Verification items for this drawing (mm, ordinates from the low corner). A direction names the side the tool comes from. Give positions to 0.01 mm unless a question says otherwise; leave off trailing zeros. Loops run counter-clockwise (first coordinate to the right, second up) from the corner with the lowest first, then second, coordinate; pieces in that order, holes last. Notation, with made-up numbers: (66, -20.75) -> (82, -20.75) arc R32 cw to (82, 13.25) -> close; hole circle Ø10 at (64.5, -32.75). An arc over 180 degrees is marked (long way). Answer as a JSON object with one key per item and string values.
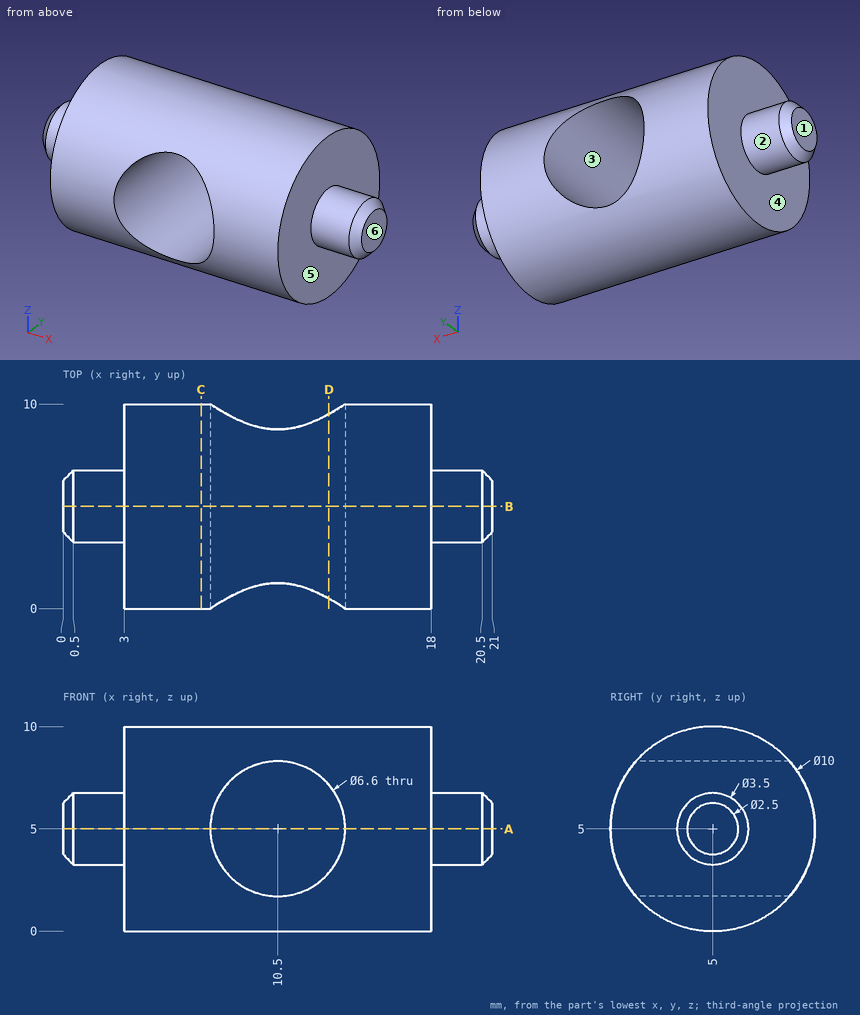
1) Section check C-C on x = 6.75. Record the cut outline in (y, z).
Geometry check:
{"outline": "circle Ø10 at (5, 5)"}
2) Draft check along Z on the marked faces 1, 2 and 3. Enter one of: pulls with the +Z half, pulls with the -Z half, needs draft (parallel to the pull), parting line crosses it, or undercut.
Geometry check:
{"face 1": "needs draft", "face 2": "parting line crosses it", "face 3": "undercut"}
3) Material ranges on line 1 along X through (y, z) = (6, 5); line 2 along X through (y, z) = (2.5, 5); line 3 along X through (y, z) = (5.25, 8.5), recorded low to high. Write a range as from..to.
Geometry check:
{"line 1": "x = 0..7.2, 13.8..21", "line 2": "x = 3..7.2, 13.8..18", "line 3": "x = 3..18"}
4) Section check D-D on x = 13. Record the cut outline in (y, z), plus the area to 3 significant figures.
Geometry check:
{"outline": "(0.49, 2.85) arc R5 ccw to (9.51, 2.85) -> close; (0.49, 7.15) -> (9.51, 7.15) arc R5 ccw to start", "area": "36.8 mm2"}
5) Section check A-A on z = 5. Record the cut outline in (x, y), plus the area to 4 significant figures.
Geometry check:
{"outline": "(0, 3.75) -> (0.5, 3.25) -> (3, 3.25) -> (3, 0) -> (7.2, 0) -> (7.2, 10) -> (3, 10) -> (3, 6.75) -> (0.5, 6.75) -> (0, 6.25) -> close; (13.8, 0) -> (18, 0) -> (18, 3.25) -> (20.5, 3.25) -> (21, 3.75) -> (21, 6.25) -> (20.5, 6.75) -> (18, 6.75) -> (18, 10) -> (13.8, 10) -> close", "area": "104.5 mm2"}
6) Tool access check on the marked faces 4, 5 and 6. Record the directions out of +Z, -Z, +X, -X, +Y, -Y that give a thin tool (end or side, any length) a straight path to the whole face; none if there is none.
Geometry check:
{"face 4": "-X", "face 5": "+X", "face 6": "+Z, -Z, +X, +Y, -Y"}
7) Depth check by flat-ended pin: P1, Ø4, axis at y = 1, z = 6, coming from the -X side; P2, Ø1.5, axis at x = 9, y = 2, coming from the +Z side; P3, Ø1, axis at x = 15, z = 2, coming from the +Y side. Enter the tip coordinate at first touch or a pass-through.
Geometry check:
{"P1": "stops at x = 3", "P2": "stops at z = 9.47", "P3": "stops at y = 9.33"}
8) Section check B-B on y = 5. Record the cut outline in (x, z).
Geometry check:
{"outline": "(0, 3.75) -> (0.5, 3.25) -> (3, 3.25) -> (3, 0) -> (18, 0) -> (18, 3.25) -> (20.5, 3.25) -> (21, 3.75) -> (21, 6.25) -> (20.5, 6.75) -> (18, 6.75) -> (18, 10) -> (3, 10) -> (3, 6.75) -> (0.5, 6.75) -> (0, 6.25) -> close; hole circle Ø6.6 at (10.5, 5)"}
